Build history of the part. All positions in model axes, mm. Round coordinates to 2 decimals unless told otherwise and drop trailing zeros. Loops run counter-clockwise (first coordinate to the right, second up) from the corner with the lowest first, then second, coordinate; pieces in that order, holes last. Notation, with made-up numbers: (-22, 20.5) - (-4, 20.5) arc R10 cw to (-4, 31.5) - close; hole circle Ø10 at (-29, 2). An arc over 180 degrees is marked (long way). Use a Markdown table: item, result.
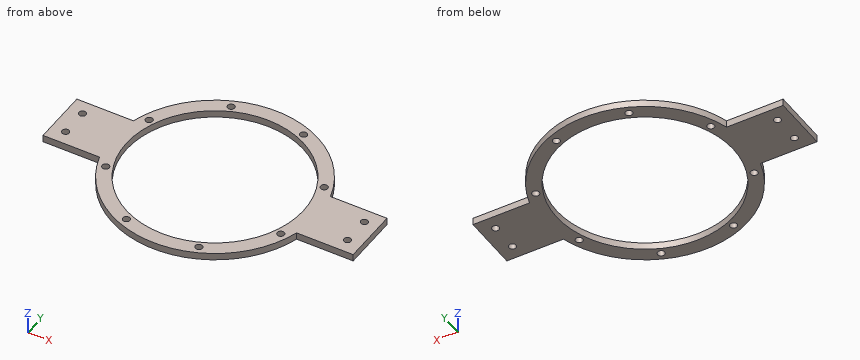
from build123d import *

# Parameters (mm, degrees)
SKETCH1_R           = 79.375
BOSS_EXTRUDE1_DEPTH = 6.35
SKETCH2_R           = 3.175
CUT_EXTRUDE1_DEPTH  = 76.2


with BuildPart() as part:
    # Sketch1 → Boss-Extrude1 (new body)
    with BuildSketch(Plane.XY):
        with BuildLine():
            Line((-139.302235141, 25.4), (-88.502235141, 25.4))
            ThreePointArc((-88.502235141, 25.4), (0, 92.075), (88.502235141, 25.4))
            Line((88.502235141, 25.4), (139.302235141, 25.4))
            Line((139.302235141, 25.4), (139.302235141, -25.4))
            Line((139.302235141, -25.4), (88.502235141, -25.4))
            ThreePointArc((88.502235141, -25.4), (0, -92.075), (-88.502235141, -25.4))
            Line((-88.502235141, -25.4), (-139.302235141, -25.4))
            Line((-139.302235141, -25.4), (-139.302235141, 25.4))
        make_face()
        Circle(SKETCH1_R, mode=Mode.SUBTRACT)
    extrude(amount=BOSS_EXTRUDE1_DEPTH)

    # Sketch2 → Cut-Extrude1 (cut)
    with BuildSketch(Plane.XY.offset(6.35)):
        with Locations((-126.602235141, -12.7)):
            Circle(SKETCH2_R)
        with Locations((-78.612909421, -32.56253326)):
            Circle(SKETCH2_R)
        with Locations((78.612909421, -32.56253326)):
            Circle(SKETCH2_R)
        with Locations((126.602235141, 12.7)):
            Circle(SKETCH2_R)
        with Locations((126.602235141, -12.7)):
            Circle(SKETCH2_R)
        with Locations((78.612909421, 32.56253326)):
            Circle(SKETCH2_R)
        with Locations((32.56253326, 78.612909421)):
            Circle(SKETCH2_R)
        with Locations((-126.602235141, 12.7)):
            Circle(SKETCH2_R)
        with Locations((-32.56253326, -78.612909421)):
            Circle(SKETCH2_R)
        with Locations((32.56253326, -78.612909421)):
            Circle(SKETCH2_R)
        with Locations((-32.56253326, 78.612909421)):
            Circle(SKETCH2_R)
        with Locations((-78.612909421, 32.56253326)):
            Circle(SKETCH2_R)
    extrude(amount=-CUT_EXTRUDE1_DEPTH, mode=Mode.SUBTRACT)


solid = part.part
Q1. Cut at A-A, the plane y = 0. List the corners of the cut face in (x, z) (3 decimals).
Results found:
| item | result |
|---|---|
| outline | (-139.302, 0) - (-79.375, 0) - (-79.375, 6.35) - (-139.302, 6.35) - close; (79.375, 0) - (139.302, 0) - (139.302, 6.35) - (79.375, 6.35) - close |
Q2. Probe line 1 (Y direction, x = -1, z = 1.25); line 2 (Y direction, x = 34, z = 0.5); line 3 (X direction, y = 1, z = 4.75). List the from-to ranges inside material, lowest first.
Results found:
| item | result |
|---|---|
| line 1 | y = -92.07 to -79.37, 79.37 to 92.07 |
| line 2 | y = -85.57 to -81.44, -75.78 to -71.72, 71.72 to 75.78, 81.44 to 85.57 |
| line 3 | x = -139.3 to -79.37, 79.37 to 139.3 |
Q3. Drop flat-ended pins along their axis: pin 1 (1 mm diameter, centred on x = 42, z = 3, fed in from +Y); pin 2 (8.5 mm diameter, centred on x = 32.56, y = -78.61, fed in from +Z). Give the stop position or say it passes through.
Results found:
| item | result |
|---|---|
| pin 1 | stops at y = 82.19 |
| pin 2 | stops at z = 6.35 |
Q4. Cut at C-C, the plane z = 4.5. Count the separate pieces of the cut face and the enclosed holes in it, plus the area to 3 significant figures.
Results found:
| item | result |
|---|---|
| separate pieces | 1 |
| enclosed holes | 13 |
| area | 11,400 mm2 |
Q5. Cut at D-D, the plane x = -102. List the corners of the cut face in (y, z).
Results found:
| item | result |
|---|---|
| outline | (-25.4, 0) - (25.4, 0) - (25.4, 6.35) - (-25.4, 6.35) - close |
Q6. Cut at B-B, the plane x = -59.5. List the corners of the cut face in (y, z).
Results found:
| item | result |
|---|---|
| outline | (-70.27, 0) - (-52.54, 0) - (-52.54, 6.35) - (-70.27, 6.35) - close; (52.54, 0) - (70.27, 0) - (70.27, 6.35) - (52.54, 6.35) - close |
